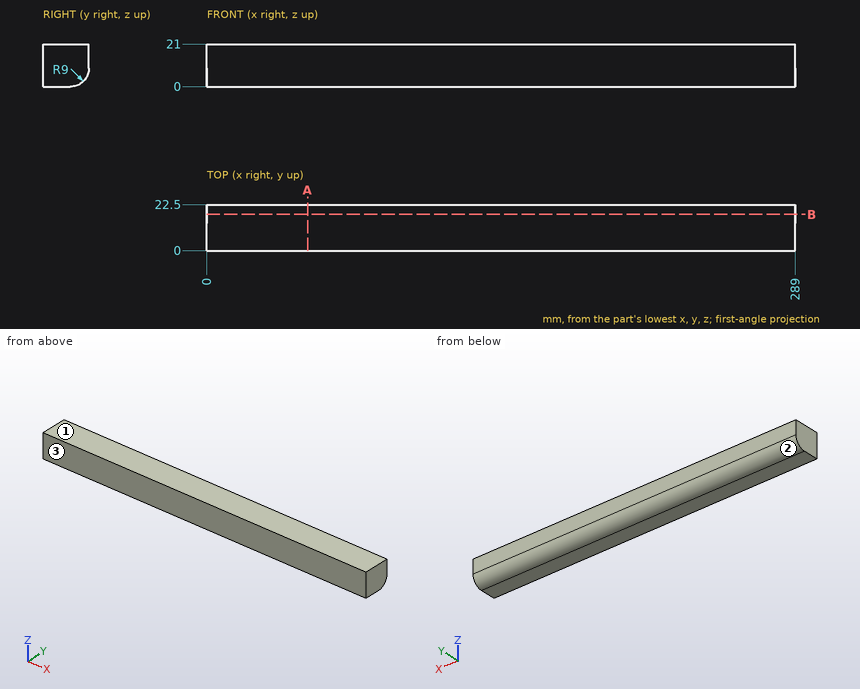
Part print with two shaded views. Sizes in mm from the minimum x, y, z corner. Round coordinates to 2 decimals unless told otherwise and drop trailing zeros. Order: outer loops, then holes, each group sorted by start corner. A loop starts at its lowest first (then second) coordinate and runs counter-clockwise, first axis right, second up. Notation, with made-up numbers: M 47,-24 L 73,-24 A24 ccw 73,13 Z; hole C 17.25,-30 d10. An arc over 180 degrees is marked long. Put each result on its own line as item: value. Start each with the question number.
1. Slice it at A-A on x = 49.5. List the corners of the cut face in (y, z), then the cut area to 3 significant figures.
2. Two-plate mould, pull along Z, no slides. Class the marked faces 1, 2 and 3: +Z half, -Z half, draft (parallel to the pull), parting line (faces both ways), or undercut.
3. Drill centre lines: probe 1 along Y at (x, z) = (177, 6.5); probe 2 along Z at (x, y) = (14, 21.25); probe 3 along Z at (x, y) = (139.5, 16). Where is each one in solid material? Low to high. Write a range as [from, to].
4. Slice it at B-B on y = 17.75. List the corners of the cut face in (x, z), then the cut area to 3 significant figures.
Findings:
1. outline: M 0,0 L 13.5,0 A9 ccw 22.5,9 L 22.5,21 L 0,21 Z
1. area: 455 mm2
2. face 1: +Z half
2. face 2: -Z half
2. face 3: draft
3. probe 1: [0, 22.15]
3. probe 2: [4.42, 21]
3. probe 3: [0.35, 21]
4. outline: M 0,1.07 L 289,1.07 L 289,21 L 0,21 Z
4. area: 5,760 mm2
